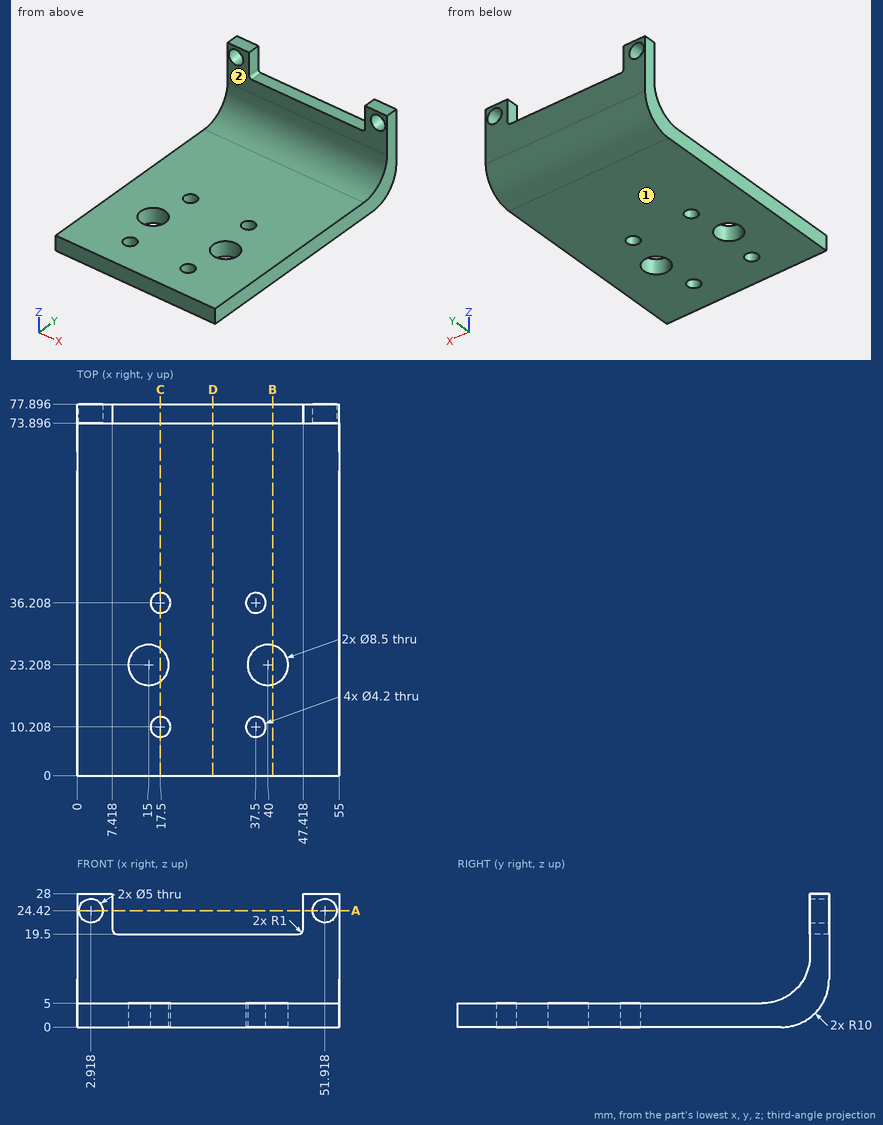
Here's the drawing with two shaded views (mm, measured from the low corner). I have some questions. A direction names the side the tool comes from. Coordinates: 2 decimals unless noted, no trailing zeros. Write each loop counter-clockwise with the first axis right and the second up, starting at its lowest first coordinate (ties: lowest second). Pieces come first, ordered by that corner, then holes. Notation, with made-up numbers: M 33.25,-6.75 L 73.25,-6.75 A22 ccw 73.25,9.25 Z; hole C 24.5,37 d4. An arc over 180 degrees is marked long. Use one line per item in the form item = value.
Q1. If we section it at D-D (x = 28.5): Write out the boundary of the cut face in (y, z).
Model answer:
outline = M 0,0 L 67.9,0 A10 ccw 77.9,10 L 77.9,19.5 L 73.9,19.5 L 73.9,15 A10 cw 63.9,5 L 0,5 Z
Q2. If we section it at A-A (z = 24.42): Write out the boundary of the cut face in (x, y), then the cut area to 3 significant figures.
Model answer:
outline = M 0,73.9 L 0.42,73.9 L 0.42,77.9 L 0,77.9 Z; M 5.42,73.9 L 7.42,73.9 L 7.42,77.9 L 5.42,77.9 Z; M 47.42,73.9 L 49.42,73.9 L 49.42,77.9 L 47.42,77.9 Z; M 54.42,73.9 L 55,73.9 L 55,77.9 L 54.42,77.9 Z
area = 20.0 mm^2
Q3. For P1, Ø2, axis at x = 37.5, y = 57.5, coming from the +Z side; P2, Ø6.5, axis at x = 32.5, z = 18.5, coming from the -Y side; P3, Ø1.2, axis at x = 33.5, y = 75, coming from the +Z side; P4, Ø12, axis at y = 70, z = 9.5, coming from the +X side, each with a flat end and sliding along its axis, tell me the tip position at first contact or that it passes through.
Model answer:
P1 = 5
P2 = 73.9
P3 = 19.5
P4 = 55
Q4. If we section it at C-C (x = 17.5): Write out the boundary of the cut face in (y, z) (1 decimal).
Model answer:
outline = M 0,0 L 8.1,0 L 8.1,5 L 0,5 Z; M 12.3,0 L 19.8,0 L 19.8,5 L 12.3,5 Z; M 26.6,0 L 34.1,0 L 34.1,5 L 26.6,5 Z; M 38.3,0 L 67.9,0 A10 ccw 77.9,10 L 77.9,19.5 L 73.9,19.5 L 73.9,15 A10 cw 63.9,5 L 38.3,5 Z
Q5. If we section it at B-B (x = 41): Write out the boundary of the cut face in (y, z), then the cut area to 3 significant figures.
Model answer:
outline = M 0,0 L 19.08,0 L 19.08,5 L 0,5 Z; M 27.34,0 L 67.9,0 A10 ccw 77.9,10 L 77.9,19.5 L 73.9,19.5 L 73.9,15 A10 cw 63.9,5 L 27.34,5 Z
area = 406 mm^2
Q6. I need wall thicknesses on line 1 along X through (y, z) = (23, 1.75) (1 decimal); line 2 along X through (y, z) = (75.7, 24.42); line 3 along Y through (x, z) = (37.5, 3.2) (1 decimal). Which ranges of each line are inside material? Lowest first, please. Write a range as from..to.
Model answer:
line_1 = 0..10.8, 19.2..35.8, 44.2..55
line_2 = 0..0.42, 5.42..7.42, 47.42..49.42, 54.42..55
line_3 = 0..8.1, 12.3..19.8, 26.6..34.1, 38.3..75.2
Q7. For the marked faces 1 and 2, which set-ups out of +Z, -Z, +X, -X, +Y, -Y let a thin tool reach every point of the face, with its end or its side?
Model answer:
face_1 = -Z, +X, -X, +Y, -Y
face_2 = +Z, +X, -X, -Y
